```python
from build123d import *

# Parameters (mm, degrees)
F5_DEPTH  = 69.9135
F7_DEPTH  = 3.98018
F9_DEPTH  = 3.26644
F10_W     = 4.318
F10_H     = 6.4389
F11_DEPTH = 25.4
F12_R     = 1.68275
F13_DEPTH = 69.9145
F16_DEPTH = 13.17344
F18_DEPTH = 13.17344


# Not quite as in the source:
# - a variable given as a bare number and used for a length is read in inches; the dataset says mm whatever the document's units were


with BuildPart() as f5:
    # F4 (on Right) → F5 (new body)
    with BuildSketch(Plane.YZ):
        Polygon((12.7127, 13.17244), (0, 11.24458), (0, 8.59028), (12.7127, 6.66242), align=None)
    extrude(amount=-F5_DEPTH)

    # F6 (on face) → F7 (join)
    with BuildSketch(Plane.YZ):
        Polygon((12.7127, 0), (12.7127, 6.66242), (0, 8.59028), (0, 0), align=None)
    extrude(amount=-F7_DEPTH)

    # F8 (on face) → F9 (join)
    with BuildSketch(Plane(origin=(-3.98018, 0, 0), x_dir=(0, -1, 0), z_dir=(-1, 0, 0))):
        Polygon((-6.4389, 7.6138314286), (-12.7127, 6.66242), (-12.7127, 0), (-6.4389, 0), align=None)
    extrude(amount=F9_DEPTH)

    # F10 (on face) → F11 (cut)
    with BuildSketch(Plane(origin=(0, 0, 0), x_dir=(1, 0, 0), z_dir=(0, 0, -1))):
        with Locations((-6.13918, -3.21945)):
            Rectangle(F10_W, F10_H)
    extrude(amount=-F11_DEPTH, mode=Mode.SUBTRACT)

    # F12 (on face) → F13 (cut, through all)
    with BuildSketch(Plane.YZ):
        with Locations((8.38835, 0)):
            Circle(F12_R)
    extrude(amount=-F13_DEPTH, mode=Mode.SUBTRACT)

    # F15 (on offset) → F16 (cut, through all)
    with BuildSketch(Plane.XY.offset(13.17244)):
        Polygon((-69.9135, 12.7127), (-69.9135, 0), (-69.0626, 12.7127), align=None)
    extrude(amount=-F16_DEPTH, mode=Mode.SUBTRACT)

    # F17 (on offset) → F18 (cut, through all)
    with BuildSketch(Plane.XY.offset(13.17244)):
        Polygon((-69.1999940296, 6.096), (-69.4737402245, 6.570142318), (-69.5177555441, 5.9125403041), align=None)
    extrude(amount=-F18_DEPTH, mode=Mode.SUBTRACT)


solid = f5.part
```
The listing builds one solid part. Answer for the finished solid, in the listing's coordinates (mm). A direction names the side the tool comes from. Give positions to 0.01 mm unless a question says otherwise; leave off trailing zeros. Write each loop counter-clockwise with the first axis right and the second up, starting at its lowest first coordinate (ties: lowest second). Pieces come first, ordered by that corner, then holes. Notation, with made-up numbers: M 38.5,81.5 L 60.5,81.5 A13 ccw 60.5,98.5 Z; hole C -14,23 d3. An arc over 180 degrees is marked long. Write each question's results on one line, items separated by ' | '.
Q1. A tool of negligible diameter and unlimited length cuts with its end or side. For faces 1 (the flat face through (-2, 3, 0)), 2 (the flat face through (-3.98, 3, 6)), 3 (the flat face through (-38.14, 6.27, 7.64)), from which of +Z, -Z, +X, -X, +Y, -Y can it reach the whole face along a straight path? Write none if from no direction.
Output values:
face 1: -Z, +X, -X, +Y, -Y | face 2: +Z, -Z, -Y | face 3: -Z, -X, -Y
Q2. Section A-A, the plane z = 9.25 is taken. Write down the section's boundary in (x, y), then the cut area to 3 significant figures.
Output values:
outline: M -69.91,0 L -8.3,0 L -8.3,6.44 L -3.98,6.44 L -3.98,0 L 0,0 L 0,12.71 L -69.06,12.71 L -69.47,6.57 L -69.2,6.1 L -69.52,5.91 Z | area: 855 mm2
Q3. Section D-D, the plane y = 9.25 is taken. Write down the section's boundary in (x, z).
Output values:
outline: M -69.29,7.19 L -7.25,7.19 L -7.25,1.45 L 0,1.45 L 0,12.65 L -69.29,12.65 Z
Q4. Section B-B, the plane y = 2.75 is taken. Write down the section's boundary in (x, z), then the cut area to 3 significant figures.
Output values:
outline: M -69.73,8.17 L -8.3,8.17 L -8.3,11.66 L -69.73,11.66 Z; M -3.98,0 L 0,0 L 0,11.66 L -3.98,11.66 Z | area: 261 mm2
Q5. For a pull along X with two mould halves and no side action, classify faces 4 (the flat face through (-6, 6.439, 6)), 5 (the flat face through (-2, 0, 6)), 6 (the flat face through (-8.298, 3, 10)), 7 (the flat face through (0, 6, 7)) as released by +X, released by -X, zero draft, split by the parting line, or undercut.
Output values:
face 4: undercut | face 5: zero draft | face 6: undercut | face 7: released by +X
Q6. Section C-C, the plane x = -10.5 is taken. Write down the section's boundary in (y, z).
Output values:
outline: M 0,8.59 L 12.71,6.66 L 12.71,13.17 L 0,11.24 Z
Q7. Flat-ended cylindrical pins translate along their axes: P1, Ø1, axis at y = 8.5, z = 4, coming from the -X side; P2, Ø1, axis at x = -29, z = 5, coming from the +Y side; P3, Ø3.5, axis at x = -6, z = 5.5, coming from the -Y side; P4, Ø6, axis at y = 2.5, z = 5, coming from the -X side. Find the tip coordinate at first contact, or state that the pin passes through.
Output values:
P1: x = -7.25 | P2: through | P3: y = 6.44 | P4: x = -3.98
Q8. Consider L1, parallel to X at y = 11, z = 5; L2, parallel to X at y = 5.25, z = 2; L3, parallel to Z at x = -52, y = 10.25. Determine where each line is inside the solid, lowest interval first. Write a range as from..to.
Output values:
L1: -7.25..0 | L2: -3.98..0 | L3: 7.04..12.8
